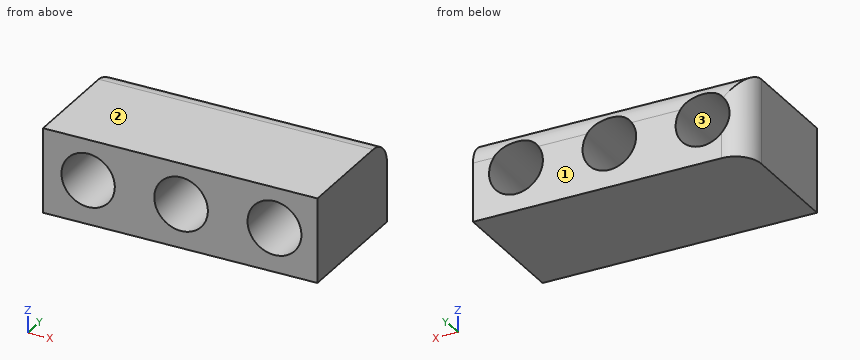
```python
from build123d import *

# Parameters (mm, degrees)
SKETCH1_W           = 21.293186277
SKETCH1_H           = 6.556248908
SKETCH1_R           = 2.09
SKETCH1_R_2         = 2.07
SKETCH1_R_3         = 2.08
BOSS_EXTRUDE1_DEPTH = 10
FILLET1_R           = 2


with BuildPart() as part:
    # Sketch1 → Boss-Extrude1 (new body)
    with BuildSketch(Plane(origin=(0, 0, 0), x_dir=(1, 0, 0), z_dir=(0, 1, 0))):
        with Locations((10.646593139, 3.278124454)):
            Rectangle(SKETCH1_W, SKETCH1_H)
        with Locations(Location((17.959518774, 3.152151811, 0), (0, 0, 270))):
            Circle(SKETCH1_R, mode=Mode.SUBTRACT)
        with Locations(Location((3.502477391, 3.152151811, 0), (0, 0, 270))):
            Circle(SKETCH1_R_2, mode=Mode.SUBTRACT)
        with Locations(Location((10.712545691, 3.152151811, 0), (0, 0, 270))):
            Circle(SKETCH1_R_3, mode=Mode.SUBTRACT)
    extrude(amount=BOSS_EXTRUDE1_DEPTH)

    # Fillet1
    # the kernel refuses this fillet: 2 mm, written as the material it takes off along each edge
    with BuildSketch(Plane(origin=(-5, 10, 0), x_dir=(0, -1, 0), z_dir=(1, 0, 0))) as fillet1_piece_1:
        with BuildLine():
            CenterArc((FILLET1_R, FILLET1_R), FILLET1_R, 180, 90)
            Line((0, FILLET1_R), (0, 0))
            Line((0, 0), (FILLET1_R, 0))
        make_face()
    extrude(amount=31.293186277, mode=Mode.SUBTRACT)
    with BuildSketch(Plane(origin=(0, 10, -11.556248908), x_dir=(0, -1, 0), z_dir=(0, 0, 1))) as fillet1_piece_2:
        with BuildLine():
            CenterArc((FILLET1_R, FILLET1_R), FILLET1_R, 180, 90)
            Line((0, FILLET1_R), (0, 0))
            Line((0, 0), (FILLET1_R, 0))
        make_face()
    extrude(amount=16.556248908, mode=Mode.SUBTRACT)


solid = part.part
```
Input: part model. Units: mm. Frame: model coordinates. Face numbers are marked on the shaded views. Round coordinates to 2 decimals unless told otherwise and drop trailing zeros. Loops run counter-clockwise (first coordinate to the right, second up) from the corner with the lowest first, then second, coordinate; pieces in that order, holes last. Notation, with made-up numbers: (-3.5, 81.25) -> (38.5, 81.25) arc R3 cw to (38.5, 86.25) -> close; hole circle Ø3 at (81.5, -4.5). An arc over 180 degrees is marked (long way). Write each question's results on one line, items separated by ' | '.
1. Mould query, pull axis Z, two halves, no side actions, for the marked faces 1, 2 and 3. Classes: +Z half, -Z half, draft (parallel to the pull), parting line (faces both ways), or undercut.
Geometry results:
face 1: draft | face 2: +Z half | face 3: undercut
2. Section B-B (x = 3). Return loops of the section in (y, z).
Geometry results:
outline: (0, -6.56) -> (10, -6.56) -> (10, -5.16) -> (0, -5.16) -> close; (0, -1.14) -> (9.81, -1.14) arc R2 ccw to (8, 0) -> (0, 0) -> close
3. Section D-D (z = -3.5). Return loops of the section in (x, y), and give its area (3 significant figures).
Geometry results:
outline: (0, 0) -> (1.46, 0) -> (1.46, 9.93) arc R2 ccw to (0, 8) -> close; (5.54, 0) -> (8.66, 0) -> (8.66, 10) -> (5.54, 10) -> close; (12.76, 0) -> (15.9, 0) -> (15.9, 10) -> (12.76, 10) -> close; (20.02, 0) -> (21.29, 0) -> (21.29, 10) -> (20.02, 10) -> close | area: 89.0 mm2
4. Ray query, line 1 (X direction, y = 7.5, z = -3); line 2 (X direction, y = 1.75, z = -5); line 3 (Z direction, x = 9.5, y = 2.75). Return the intervals inside material, ascending. Write a range as from..to.
Geometry results:
line 1: 0..1.44, 5.57..8.64, 12.79..15.88, 20.04..21.29 | line 2: 0..2.57, 4.44..9.76, 11.67..16.98, 18.94..21.29 | line 3: -6.56..-4.84, -1.46..0
5. Section C-C (y = 8.5). Return loops of the section in (x, z).
Geometry results:
outline: (0.06, -6.56) -> (21.29, -6.56) -> (21.29, -0.06) -> (0.06, -0.06) -> close; hole circle Ø4.14 at (3.5, -3.15); hole circle Ø4.16 at (10.71, -3.15); hole circle Ø4.18 at (17.96, -3.15)
6. Section A-A (z = -2.5). Return loops of the section in (x, y), and give its area (3 significant figures).
Geometry results:
outline: (0, 0) -> (1.54, 0) -> (1.54, 9.95) arc R2 ccw to (0, 8) -> close; (5.47, 0) -> (8.74, 0) -> (8.74, 10) -> (5.47, 10) -> close; (12.69, 0) -> (15.97, 0) -> (15.97, 10) -> (12.69, 10) -> close; (19.95, 0) -> (21.29, 0) -> (21.29, 10) -> (19.95, 10) -> close | area: 93.6 mm2
